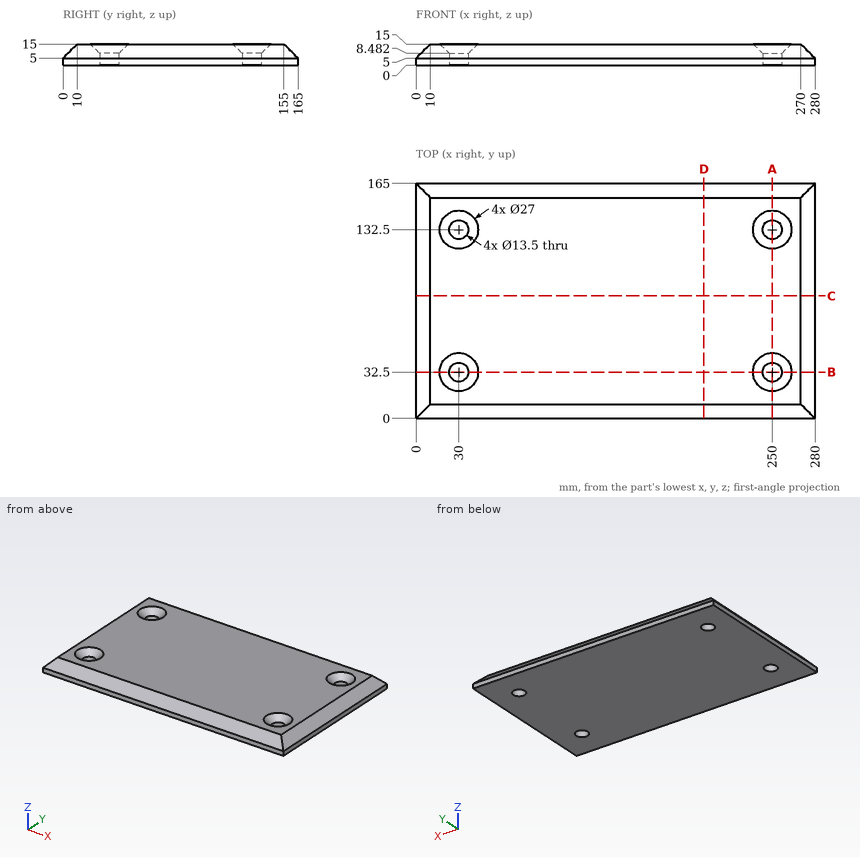
Job drawing, mm, ordinate dimensions from the low corner. One solid piece. Give positions to 0.01 mm unless a question says otherwise; leave off trailing zeros. Order: outer loops, then holes, each group sorted by start corner. A loop starts at its lowest first (then second) coordinate and runs counter-clockwise, first axis right, second up. Notation, with made-up numbers: (6.25, 78) - (25.25, 78) arc R32 cw to (25.25, 104) - close; hole circle Ø10 at (32, -5.5). An arc over 180 degrees is marked (long way). One line per question, with ' | ' between items.
1. Drop flat-ended pins along their axis: P1, Ø12, axis at x = 30, y = 132.5, coming from the +Z side; P2, Ø21.5, axis at x = 30, y = 32.5, coming from the +Z side (1 decimal); P3, Ø5, axis at x = 203.5, y = 72.5, coming from the -Z side; P4, Ø1.5, axis at y = 93, z = 12.5, coming from the -X side. Give the stop position or say it passes through.
Filled in:
P1: through | P2: z = 12.3 | P3: z = 0 | P4: x = 6.75
2. Band-saw the part on A-A on x = 250. List the corners of the cut face in (y, z).
Filled in:
outline: (0, 0) - (25.75, 0) - (25.75, 8.48) - (19, 15) - (10, 15) - (0, 5) - close; (39.25, 0) - (125.75, 0) - (125.75, 8.48) - (119, 15) - (46, 15) - (39.25, 8.48) - close; (139.25, 0) - (165, 0) - (165, 5) - (155, 15) - (146, 15) - (139.25, 8.48) - close
3. Band-saw the part on D-D on x = 202. List the corners of the cut face in (y, z).
Filled in:
outline: (0, 0) - (165, 0) - (165, 5) - (155, 15) - (10, 15) - (0, 5) - close
4. Band-saw the part on B-B on y = 32.5. List the corners of the cut face in (x, z).
Filled in:
outline: (0, 0) - (23.25, 0) - (23.25, 8.48) - (16.5, 15) - (10, 15) - (0, 5) - close; (36.75, 0) - (243.25, 0) - (243.25, 8.48) - (236.5, 15) - (43.5, 15) - (36.75, 8.48) - close; (256.75, 0) - (280, 0) - (280, 5) - (270, 15) - (263.5, 15) - (256.75, 8.48) - close
5. Drill centre lines: probe 1 along Y at (x, z) = (250, 2.5); probe 2 along X at (y, z) = (132.5, 2); probe 3 along Y at (x, z) = (23, 10.5). Where is each one in solid material? Low to high.
Filled in:
probe 1: 0 to 25.75, 39.25 to 125.75, 139.25 to 165 | probe 2: 0 to 23.25, 36.75 to 243.25, 256.75 to 280 | probe 3: 5.5 to 27.1, 37.9 to 127.1, 137.9 to 159.5
6. Band-saw the part on C-C on y = 86. List the corners of the cut face in (x, z), then the cut area to 3 significant figures.
Filled in:
outline: (0, 0) - (280, 0) - (280, 5) - (270, 15) - (10, 15) - (0, 5) - close | area: 4,100 mm²
